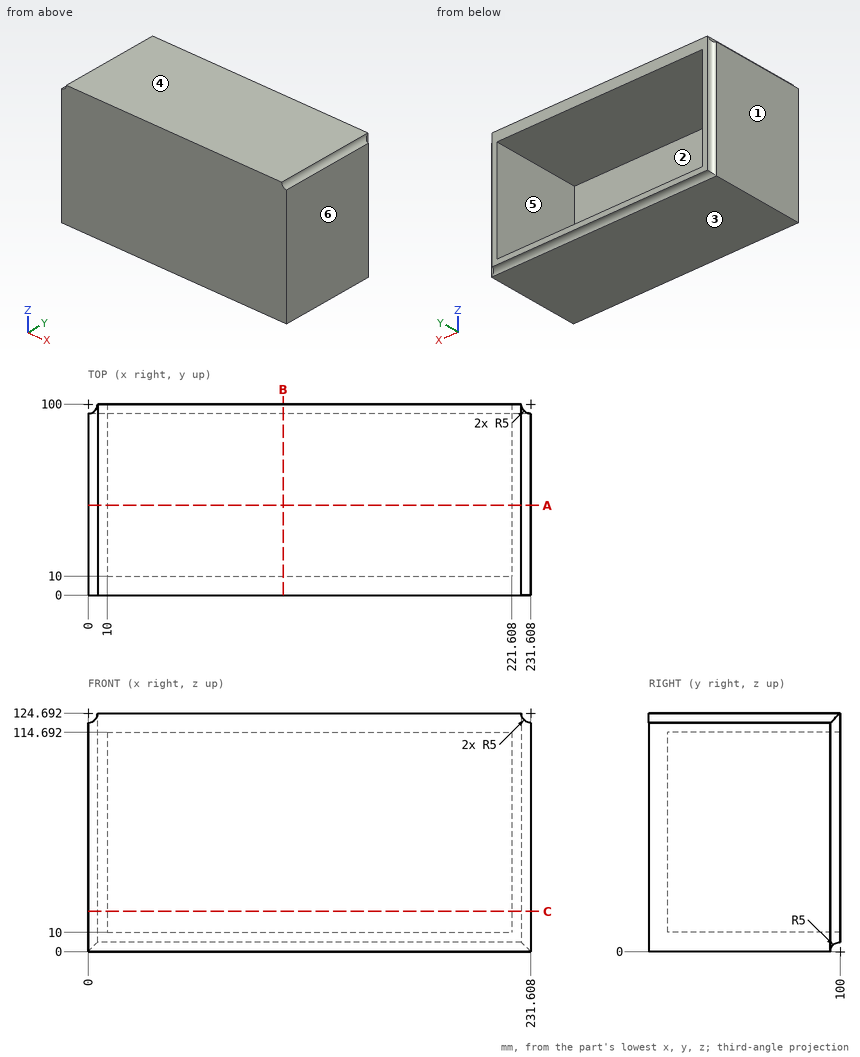
Study the drawing (mm; zero at the part's minimum x, y, z) and answer. A direction names the side the tool comes from. Give positions to 0.01 mm unless a question says otherwise; leave off trailing zeros. Loops run counter-clockwise (first coordinate to the right, second up) from the corner with the lowest first, then second, coordinate; pieces in that order, holes last. Notation, with made-up numbers: (45, -24.5) - (64, -24.5) arc R25 ccw to (64, -2.5) - close; hole circle Ø7 at (50.25, 83.25). An arc over 180 degrees is marked (long way). Answer as CSV lines item,"result". Start each with the question number.
1) Straight lines are drawn through the part: L1, parallel to X at y = 85.5, z = 72.5; L2, parallel to Z at x = 183.5, y = 63; L3, parallel to Y at x = 116, z = 38. For each, find the intervals that lie inside material, in ascending order. Write a range as from..to.
2) Find section B-B (x = 102). Write down the section's boundary in (y, z), then the cut area to 3 significant figures.
3) Find section A-A (y = 47). Write down the section's boundary in (x, z).
4) Find section C-C (z = 21). Write down the section's boundary in (x, y).
5) This flat-tipped pin is pushed along its axis until it touches: pin 1 Ø2 at (x, z) = (168.5, 43.5) entering from -Y. Where does it stop, or does it pass through?
6) Determine the mould class of the marked faces 1, 2, 3 and 4 for opening direction Z: released by +Z, released by -Z, zero draft, split by the parting line, or undercut.
7) Which of the six approach directions +Z, -Z, +X, -X, +Y, -Y give full straight-line access (tool end or side, diameter ignored) to the marked faces 5 and 6?
Findings below:
1,L1,"0..10, 221.61..231.61"
1,L2,"0..10, 114.69..124.69"
1,L3,"0..10"
2,outline,"(0, 0) - (95, 0) arc R5 cw to (100, 5) - (100, 10) - (10, 10) - (10, 114.69) - (100, 114.69) - (100, 124.69) - (0, 124.69) - close"
2,area,"3,030 mm^2"
3,outline,"(0, 0) - (231.61, 0) - (231.61, 119.69) arc R5 cw to (226.61, 124.69) - (5, 124.69) arc R5 cw to (0, 119.69) - close; hole (10, 10) - (221.61, 10) - (221.61, 114.69) - (10, 114.69) - close"
4,outline,"(0, 0) - (231.61, 0) - (231.61, 95) arc R5 cw to (226.61, 100) - (221.61, 100) - (221.61, 10) - (10, 10) - (10, 100) - (5, 100) arc R5 cw to (0, 95) - close"
5,pin 1,"y = 0"
6,face 1,"zero draft"
6,face 2,"undercut"
6,face 3,"released by -Z"
6,face 4,"released by +Z"
7,face 5,"+Y"
7,face 6,"+Z, -Z, +X, +Y, -Y"
